from build123d import *

# Parameters (mm, degrees)
F0_W     = 210
F0_H     = 40
F1_DEPTH = 9
F2_D     = 10
F3_R     = 7.5


with BuildPart() as f1:
    # F0 (on Top) → F1 (new body)
    with BuildSketch(Plane.XY):
        with Locations((0, 2.5)):
            Rectangle(F0_W, F0_H)
    extrude(amount=F1_DEPTH)

    # F2 (through all)
    with Locations(Plane(origin=(0, 0, 0), x_dir=(1, 0, 0), z_dir=(0, 0, -1))):
        with Locations((-95, 0.5), (-7.5, -1.5), (85, -4)):
            Hole(F2_D / 2)

    # F3
    f3_edges = [f1.edges().sort_by_distance(p)[0] for p in [
        (-105, 22.5, 4.5),
        (-105, -17.5, 4.5),
        (105, 22.5, 4.5),
        (105, -17.5, 4.5),
    ]]
    fillet(f3_edges, radius=F3_R)


solid = f1.part
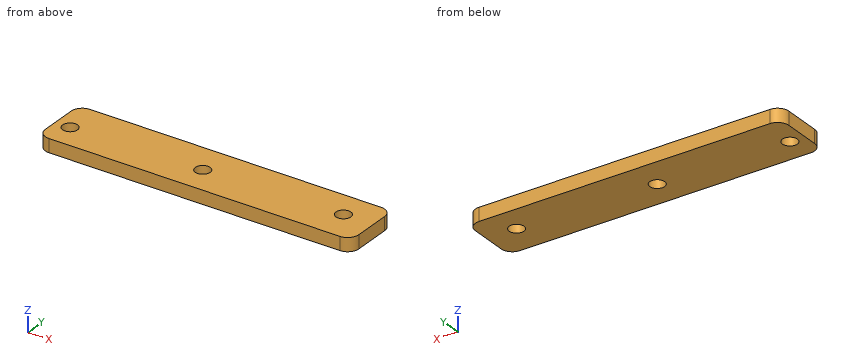
Geometry: final body of the model. Coordinates: model frame, mm. Give positions to 0.01 mm unless a question says otherwise; leave off trailing zeros. Write each loop counter-clockwise with the first axis right and the second up, starting at its lowest first coordinate (ties: lowest second). Pieces come first, ordered by that corner, then holes. Notation, with made-up numbers: M 70.5,48 L 98.5,48 A18 cw 98.5,74 Z; hole C -35.75,-12 d3. An arc over 180 degrees is marked long. Answer in a Markdown table with one row per item. Add a question column.
(1) Section B-B on x = -7.5. Return loops of the section in (y, z).
(2) Ray query, line 1 (Y direction, x = -7.5, z = 3); line 2 (Y direction, x = -95, z = 3.25); line 3 (X direction, y = -12, z = 2.5). Return the intervals inside material, ascending.
(3) Section A-A on z = 6. Return loops of the section in (x, y), and give its area (3 significant figures).
Result set:
| question | item | result |
|---|---|---|
| 1 | outline | M -17.5,0 L -3.5,0 L -3.5,9 L -17.5,9 Z; M 6.5,0 L 22.5,0 L 22.5,9 L 6.5,9 Z |
| 2 | line 1 | y = -17.5 to -3.5, 6.5 to 22.5 |
| 2 | line 2 | y = -17.5 to -5.5, 4.5 to 22.5 |
| 2 | line 3 | x = -104.73 to 104.73 |
| 3 | outline | M -105,-10 A7.5 ccw -97.5,-17.5 L 97.5,-17.5 A7.5 ccw 105,-10 L 105,15 A7.5 ccw 97.5,22.5 L -97.5,22.5 A7.5 ccw -105,15 Z; hole C -95,-0.5 d10; hole C -7.5,1.5 d10; hole C 85,4 d10 |
| 3 | area | 8,120 mm^2 |
